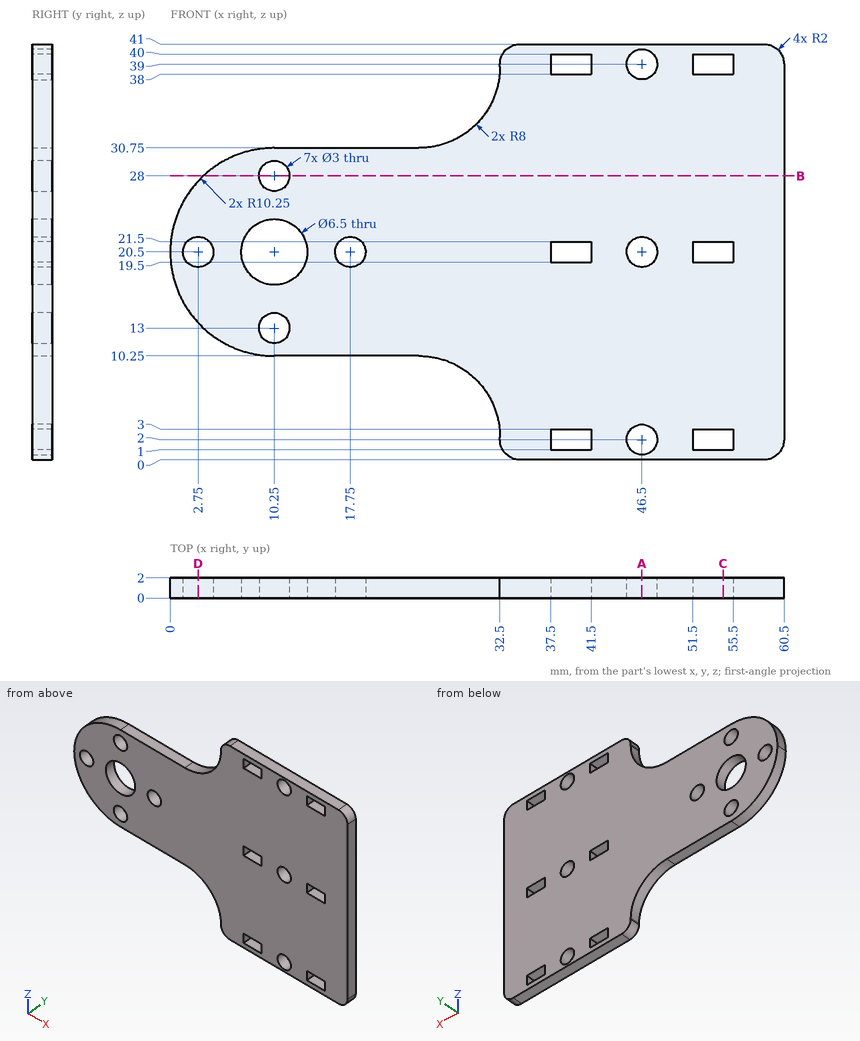
Geometry check sheet. Reference: drawing and pictorial views, mm from the part's lowest x, y, z. Give positions to 0.01 mm unless a question says otherwise; leave off trailing zeros. Write each loop counter-clockwise with the first axis right and the second up, starting at its lowest first coordinate (ties: lowest second). Pieces come first, ordered by that corner, then holes.
Item 1: Scan lines: L1, parallel to Z at x = 55, y = 1.3; L2, parallel to Z at x = 47, y = 1.65; L3, parallel to X at y = 0.4, z = 39.5. Record each from-to range of solid material in increasing order.
Item 2: Cross-section at B-B (z = 28). Enter the section's corners in (x, y).
Item 3: Cross-section at C-C (x = 54.5). Enter the section's corners in (y, z).
Item 4: Cross-section at A-A (x = 46.5). Enter the section's corners in (y, z), and give its area (3 significant figures).
Item 5: Gauge pin test, flat end, axial feed: pin 1 (2 mm diameter, centred on x = 6.5, z = 8.5, fed in from -Y). Record the tip position at first contact, or that the pin passes through.
Item 6: Cross-section at D-D (x = 2.75). Enter the section's corners in (y, z).
Report:
1. L1: z = 0 to 1, 3 to 19.5, 21.5 to 38, 40 to 41
1. L2: z = 0 to 0.59, 3.41 to 19.09, 21.91 to 37.59, 40.41 to 41
1. L3: x = 32.56 to 37.5, 41.5 to 45.09, 47.91 to 51.5, 55.5 to 60.44
2. outline: (3.26, 0) - (8.75, 0) - (8.75, 2) - (3.26, 2) - close; (11.75, 0) - (60.5, 0) - (60.5, 2) - (11.75, 2) - close
3. outline: (0, 0) - (2, 0) - (2, 1) - (0, 1) - close; (0, 3) - (2, 3) - (2, 19.5) - (0, 19.5) - close; (0, 21.5) - (2, 21.5) - (2, 38) - (0, 38) - close; (0, 40) - (2, 40) - (2, 41) - (0, 41) - close
4. outline: (0, 0) - (2, 0) - (2, 0.5) - (0, 0.5) - close; (0, 3.5) - (2, 3.5) - (2, 19) - (0, 19) - close; (0, 22) - (2, 22) - (2, 37.5) - (0, 37.5) - close; (0, 40.5) - (2, 40.5) - (2, 41) - (0, 41) - close
4. area: 64.0 mm2
5. pin 1: passes through
6. outline: (0, 13.51) - (2, 13.51) - (2, 19) - (0, 19) - close; (0, 22) - (2, 22) - (2, 27.49) - (0, 27.49) - close
